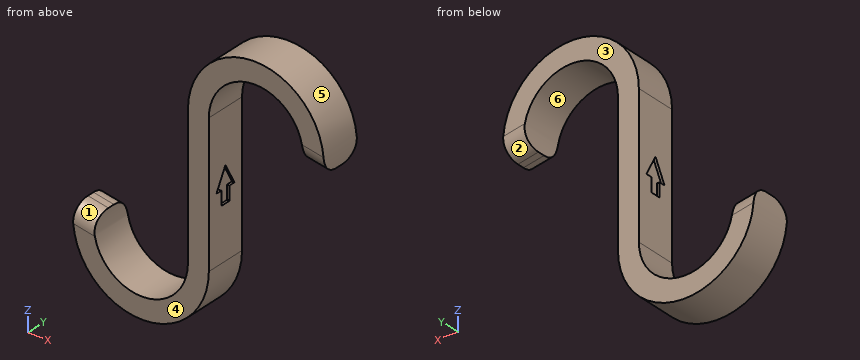
from build123d import *

# Parameters (mm, degrees)
SKETCH003_W       = 6
SKETCH003_H       = 12
POCKET_DEPTH      = 36.001
POCKET_DEPTH_BACK = 36.001
FILLET_R          = 5
PAD_DEPTH         = 2.3


with BuildPart() as part:
    # AdditivePipe: sweep along a path in Sketch
    with BuildLine(Plane.XZ) as additivepipe_path:
        ThreePointArc((-32.749328, -17.134805), (-17.93807, -36.437213), (0, -20))
        Line((0, -20), (0, 20))
        ThreePointArc((0, 20), (17.93807, 36.437213), (32.749328, 17.134805))
    # Sketch003 → AdditivePipe (sweep)
    with BuildSketch(Plane.XY):
        Rectangle(SKETCH003_W, SKETCH003_H)
    sweep(path=additivepipe_path.line)

    # Sketch002 → Pocket (cut, two sides)
    with BuildSketch(Plane.YZ) as pocket_sk:
        Polygon((3.25, -1), (0, 5), (-3.25, -1), (-1.5, -1), (-1.5, -5), (1.5, -5), (1.5, -1), align=None)
    extrude(amount=-POCKET_DEPTH, mode=Mode.SUBTRACT)
    extrude(pocket_sk.sketch, amount=POCKET_DEPTH_BACK, mode=Mode.SUBTRACT)

    # Fillet
    fillet_edges = [part.edges().sort_by_distance(p)[0] for p in [
        (32.749328, 6, 17.134805),
        (32.749328, -6, 17.134805),
        (-32.749328, -6, -17.134805),
        (-32.749328, 6, -17.134805),
    ]]
    fillet(fillet_edges, radius=FILLET_R)

    # Sketch002 → Pad (join, symmetric)
    with BuildSketch(Plane.YZ):
        Polygon((3.25, -1), (0, 5), (-3.25, -1), (-1.5, -1), (-1.5, -5), (1.5, -5), (1.5, -1), align=None)
    extrude(amount=PAD_DEPTH, both=True)


solid = part.part
Geometry: final body of the model. Coordinates: model frame, mm. Face numbers are marked on the shaded views. A direction names the side the tool comes from. Round coordinates to 2 decimals unless told otherwise and drop trailing zeros. Loops run counter-clockwise (first coordinate to the right, second up) from the corner with the lowest first, then second, coordinate; pieces in that order, holes last.
Q1. Section C-C on x = -16.5. Return loops of the section in (y, z).
Q2. Access query for the marked faces 1, 2 and 3. Directions: +Z, -Z, +X, -X, +Y, -Y. A direction counts if a zero-diameter tool reaches every point of the face in a straight line with its end or side. Return the directions, or none.
Q3. Pull-direction query (X, two-part tool) for the marked faces 4, 5 and 6; classes: released by +X, released by -X, zero draft, split by the parting line, or undercut.
Q4. Pin query (flat end, axial travel): P1, Ø0.6, axis at x = 2.5, y = 0.5, coming from the +Z side; P2, Ø1.5, axis at y = 2.5, z = -25.5, coming from the +X side; P3, Ø2, axis at y = 1, z = -1.5, coming from the -X side; P4, Ø24.5, axis at x = 16.5, z = 20, coming from the -Y side. Return the tip coordinate at first contact, or that it passes through.
Q5. Section B-B on z = 11. Return loops of the section in (x, y), plus the area to 3 significant figures.
Q6. Material intervals for L1, parallel to X at y = -3, z = 20; L2, parallel to X at y = 0, z = -20; L3, parallel to Z at x = 16.5, y = -3.5, sorted ascending.
Evaluation:
1. outline: (-6, -39.5) - (6, -39.5) - (6, -33.5) - (-6, -33.5) - close
2. face 1: +Z, -Y
2. face 2: -Z, +Y
2. face 3: +Z, -Z, +X, -X, +Y
3. face 4: zero draft
3. face 5: split by the parting line
3. face 6: undercut
4. P1: stops at z = 33.88
4. P2: stops at x = 2.41
4. P3: stops at x = -3
4. P4: passes through
5. outline: (-3, -6) - (3, -6) - (3, 6) - (-3, 6) - close
5. area: 72.0 mm2
6. L1: x = -3 to 3, 30 to 36
6. L2: x = -36 to -30, -3 to 3
6. L3: z = 33.5 to 39.5
